Autodesk Inventor part; units mm, degrees
ref_plane "YZ Plane" through (0, 0, 0) normal (1, 0, 0) x (0, 1, 0)
ref_plane "XZ Plane" through (0, 0, 0) normal (0, 1, 0) x (-1, 0, 0)
ref_plane "XY Plane" through (0, 0, 0) normal (0, 0, 1) x (1, 0, 0)
sketch "Skizze1" plane through (0, 0, 0) normal (0, 0, 1) x (1, 0, 0)
  line L0 (-6.5297, -2.8796) -> (43.4703, -2.8796)
  line L1 (43.4703, -2.8796) -> (43.4703, 8.1204)
  line L2 (43.4703, 8.1204) -> (-6.5297, 8.1204)
  line L3 (-6.5297, 8.1204) -> (-6.5297, -2.8796)
  point P0 (0, 0)
  dimension "d0" = 50
  dimension "d1" = 11
extrude "Extrusion1" add sketch "Skizze1" along normal blind 7
sketch "Skizze2" plane through (-6.5297, 8.1204, 0) normal (0, 1, 0) x (1, 0, 0)
  line L0 (29.65, -5.55) -> (20.35, -5.55)
  line L1 (20.35, -5.55) -> (20.35, -1.45)
  line L2 (20.35, -1.45) -> (29.65, -1.45)
  line L3 (29.65, -1.45) -> (29.65, -5.55)
  line L4 (50, -7) -> (0, -7)
  line L5 (50, 0) -> (50, -7)
  line L6 (0, 0) -> (0, -7)
  point P0 (6.5297, 0)
  dimension "d4" = 9.3
  dimension "d5" = 4.1
  dimension "d6" = 1.45
  dimension "d7" = 20.35
  dimension "d8" = 20.35
extrude "Extrusion2" cut sketch "Skizze2" against normal blind 9.35
sketch "Skizze3" plane through (0, 0, 7) normal (0, 0, 1) x (1, 0, 0)
  line L0 (-6.5297, 8.1204) -> (-6.5297, -2.8796)
  line L1 (43.4703, 8.1204) -> (-6.5297, 8.1204)
  point P0 (0, 0)
  point P1 (5.9703, 2.2704)
  point P2 (18.4703, 2.2704)
  point P3 (30.9703, 2.2704)
  dimension "d11" = 12.5
  dimension "d12" = 12.5
  dimension "d13" = 12.5
  dimension "d14" = 5.85
hole "Bohrung1" at (5.9703, 2.2704, 7) at (18.4703, 2.2704, 7) at (30.9703, 2.2704, 7) direction (0, 0, -1) diameter 6.15 end through all
sketch "Skizze4" plane through (-6.5297, 8.1204, 0) normal (0, 1, 0) x (1, 0, 0)
  point P0 (6.5297, 0)
sketch "Skizze5" plane through (-6.5297, 8.1204, 0) normal (0, 1, 0) x (1, 0, 0)
  line L0 (50, 0) -> (0, 0)
  line L1 (0, 0) -> (0, -53.0037)
  line L2 (0, -53) -> (50, -53)
  line L3 (50, -53) -> (50, 46)
  line L4 (50, 46) -> (0, 46)
  line L5 (0, 46) -> (0, -53)
  point P0 (6.5297, 0)
  dimension "d22" = 50
  dimension "d23" = 99
  dimension "d24" = 46
extrude "Extrusion3" add sketch "Skizze5" along normal blind 3.5
sketch "Skizze6" plane through (-6.5297, 11.6204, 0) normal (0, 1, 0) x (1, 0, 0)
  line L0 (29.65, -1.45) -> (29.65, -5.55)
  line L1 (29.65, -1.45) -> (20.35, -1.45)
  line L2 (20.35, -1.45) -> (20.35, -5.55)
  line L3 (20.35, -5.55) -> (29.65, -5.55)
  line L4 (29.65, -5.55) -> (29.65, -1.45)
  point P0 (6.5297, 0)
extrude "Extrusion4" cut sketch "Skizze6" against normal blind 3.5
sketch "Skizze7" plane through (-6.5297, 11.6204, 0) normal (0, 1, 0) x (1, 0, 0)
  line L0 (0, -53) -> (50, -53)
  line L1 (50, -53) -> (42.5, -53)
  line L2 (42.5, -53) -> (42.5, -42.5)
  line L3 (42.5, -42.5) -> (50, -42.5)
  line L4 (50, -42.5) -> (50, -53)
  line L5 (0, -53) -> (7.5, -53)
  line L6 (7.5, -53) -> (7.5, -42.5)
  line L7 (7.5, -42.5) -> (0, -42.5)
  line L8 (0, -42.5) -> (0, -53)
  line L9 (0, 46) -> (0, -53)
  line L10 (0, 46) -> (7.5, 46)
  line L11 (7.5, 46) -> (7.5, 35.5)
  line L12 (7.5, 35.5) -> (0, 35.5)
  line L13 (0, 35.5) -> (0, 46)
  line L14 (50, -53) -> (50, 46)
  line L15 (50, 46) -> (42.5, 46)
  line L16 (42.5, 46) -> (42.5, 35.5)
  line L17 (42.5, 35.5) -> (50, 35.5)
  line L18 (50, 35.5) -> (50, 46)
  point P0 (6.5297, 0)
  dimension "d29" = 7.5
  dimension "d30" = 10.5
  dimension "d31" = 7.5
  dimension "d32" = 10.5
  dimension "d33" = 7.5
  dimension "d34" = 10.5
  dimension "d35" = 7.5
  dimension "d36" = 10.5
extrude "Extrusion5" add sketch "Skizze7" along normal blind 25
sketch "Skizze8" plane through (0.9703, 11.6204, -35.5) normal (1, 0, 0) x (0, 0, -1)
  point P0 (-35.5, -11.6204)
sketch "Skizze9" plane through (-6.5297, 36.6204, 0) normal (0, 1, 0) x (1, 0, 0)
  line L0 (50, -42.5) -> (50, 35.5)
  line L1 (0, 46) -> (50, 46)
  line L2 (50, 46) -> (50, 35.5)
  line L3 (50, 35.5) -> (0, 35.5)
  line L4 (0, 35.5) -> (0, 46)
  line L5 (50, -53) -> (50, -7)
  line L6 (0, -42.5) -> (50, -42.5)
  line L7 (50, -42.5) -> (50, -53)
  line L8 (50, -53) -> (0, -53)
  line L9 (0, -53) -> (0, -42.5)
  line L10 (50, -42.5) -> (42.5, -42.5)
  point P0 (6.5297, 0)
  dimension "d75" = 0
extrude "Extrusion6" add sketch "Skizze9" along normal blind 5
sketch "Skizze10" plane through (-6.5297, 41.6204, 0) normal (0, 1, 0) x (1, 0, 0)
  line L0 (50, 46) -> (0, 46)
  line L1 (0, -53) -> (50, -53)
  line L2 (42.5, -42.5) -> (42.5, -53)
  line L3 (42.5, 46) -> (42.5, 35.5)
  line L4 (7.5, 35.5) -> (7.5, 46)
  line L5 (7.5, -53) -> (7.5, -42.5)
  point P0 (6.5297, 0)
  point P1 (15.7518, 40.75)
  point P2 (25, 40.75)
  point P3 (33.5, 40.75)
  point P4 (15.6745, -47.75)
  point P5 (25, -47.75)
  point P6 (33.5, -47.75)
  dimension "d41" = 5.25
  dimension "d42" = 5.25
  dimension "d43" = 5.25
  dimension "d44" = 5.25
  dimension "d45" = 5.25
  dimension "d46" = 5.25
  dimension "d47" = 9
  dimension "d50" = 9
  dimension "d76" = 17.5
  dimension "d77" = 17.5
hole "Bohrung2" at (18.4703, 41.6204, 47.75) at (18.4703, 41.6204, -40.75) direction (0, -1, 0) diameter 6 depth 10 tip angle 118
sketch "Skizze11" plane through (-6.5297, 41.6204, 0) normal (0, 1, 0) x (1, 0, 0)
  line L0 (7.5, -53) -> (7.5, -42.5)
  line L1 (42.5, -42.5) -> (42.5, -53)
  line L2 (50, -42.5) -> (0, -42.5)
  line L3 (50, 46) -> (0, 46)
  line L4 (42.5, 46) -> (42.5, 35.5)
  line L5 (7.5, 35.5) -> (7.5, 46)
  point P0 (6.5297, 0)
  point P1 (16.5, -47.75)
  point P2 (33.5, -47.75)
  point P3 (16.5, 40.75)
  point P4 (33.5, 40.75)
  dimension "d60" = 9
  dimension "d61" = 9
  dimension "d62" = 5.25
  dimension "d63" = 5.25
  dimension "d64" = 5.25
  dimension "d65" = 5.25
  dimension "d66" = 9
  dimension "d67" = 9
hole "Bohrung3" at (9.9703, 41.6204, 47.75) at (26.9703, 41.6204, 47.75) at (9.9703, 41.6204, -40.75) at (26.9703, 41.6204, -40.75) direction (0, -1, 0) diameter 6.2 depth 31.5 tip angle 118
sketch "Skizze12" plane through (-6.5297, -2.8796, 0) normal (0, -1, 0) x (1, 0, 0)
  point P0 (6.5297, 0)
properties part number "Objektträgerhalter 1 Neu"
Geometry check sheet. Reference: the model listing, model coordinates, mm. A direction names the side the tool comes from. Round coordinates to 2 decimals unless told otherwise and drop trailing zeros. Loops run counter-clockwise (first coordinate to the right, second up) from the corner with the lowest first, then second, coordinate; pieces in that order, holes last. Notation, with made-up numbers: (25, 14) - (66, 14) arc R15 cw to (66, 28) - close; hole circle Ø11 at (29.5, 39). An arc over 180 degrees is marked (long way). One line per question, with ' | ' between items. Start each with the question number.
1. Scan lines: line 1 (X direction, y = 38, z = 47.75); line 2 (Z direction, x = -1, y = 28); line 3 (X direction, y = 21.5, z = 43.5). Record each from-to range of solid material in increasing order. Write a range as [from, to].
2. Draft check along Z on faces 6 (the face through (43.47, 11, 4)), 7 (the face through (18.338, 39.085, 44.753)), 8 (the face through (18, 6, 7)). Enter one of: released by +Z, released by -Z, zero draft, split by the parting line, or undercut.
3. Cross-section at C-C on y = 38. Record the cut outline in (x, z).
4. Cross-section at B-B on x = 4.5. Record the cut outline in (y, z), then the cut area to 3 significant figures.
5. Tool access check on faces 1 (the face through (-6.53, 11, 3)), 2 (the face through (11.158, 39.085, -37.886)), 3 (the face through (0.97, 24, -41)), 4 (the face through (18, 6, 0)), 5 (the face through (18, 38, 42.5)). Record the directions out of +Z, -Z, +X, -X, +Y, -Y that give a thin tool (end or side, any length) a straight path to the whole face; none if there is none.
6. Cross-section at A-A on y = 30. Record the cut outline in (x, z), then the cut area to 3 significant figures.
7. Depth check by flat-ended pin: pin 1 (3.5 mm diameter, centred on x = 18.5, z = 3, fed in from +Y); pin 2 (8.5 mm diameter, centred on x = 25, z = -39.5, fed in from -Y); pin 3 (5.5 mm diameter, centred on x = 10, y = 1, fed in from +Z). Enter the tip coordinate at first touch or a pass-through.
8. Cross-section at D-D on x = 17.5. State how many separate pieces and enclosed holes the cut face has, then the cut area to 3 significant figures.
Taken from the geometry:
1) line 1: [-6.53, 6.87], [13.07, 15.47], [21.47, 23.87], [30.07, 43.47] | line 2: [-46, -35.5], [42.5, 53] | line 3: [-6.53, 0.97], [35.97, 43.47]
2) face 6: zero draft | face 7: undercut | face 8: released by +Z
3) outline: (-6.53, -46) - (43.47, -46) - (43.47, -35.5) - (-6.53, -35.5) - close; (-6.53, 42.5) - (43.47, 42.5) - (43.47, 53) - (-6.53, 53) - close; hole circle Ø6.2 at (9.97, -40.75); hole circle Ø6.2 at (9.97, 47.75); hole circle Ø6 at (18.47, -40.75); hole circle Ø6 at (18.47, 47.75); hole circle Ø6.2 at (26.97, -40.75); hole circle Ø6.2 at (26.97, 47.75)
4) outline: (-2.88, 0) - (-0.43, 0) - (-0.43, 7) - (-2.88, 7) - close; (4.97, 0) - (8.12, 0) - (8.12, -46) - (11.62, -46) - (11.62, 53) - (8.12, 53) - (8.12, 7) - (4.97, 7) - close; (36.62, -46) - (41.62, -46) - (41.62, -35.5) - (36.62, -35.5) - close; (36.62, 42.5) - (41.62, 42.5) - (41.62, 53) - (36.62, 53) - close | area: 491 mm²
5) face 1: +Z, -Z, -X, +Y, -Y | face 2: +Y | face 3: +Z, -Z | face 4: -Z, +X, -X, -Y | face 5: +X, -X, +Y
6) outline: (-6.53, -46) - (0.97, -46) - (0.97, -35.5) - (-6.53, -35.5) - close; (-6.53, 42.5) - (0.97, 42.5) - (0.97, 53) - (-6.53, 53) - close; (35.97, -46) - (43.47, -46) - (43.47, -35.5) - (35.97, -35.5) - close; (35.97, 42.5) - (43.47, 42.5) - (43.47, 53) - (35.97, 53) - close | area: 315 mm²
7) pin 1: y = 11.62 | pin 2: y = 8.12 | pin 3: z = 7
8) separate pieces: 7 | enclosed holes: 0 | area: 402 mm²
